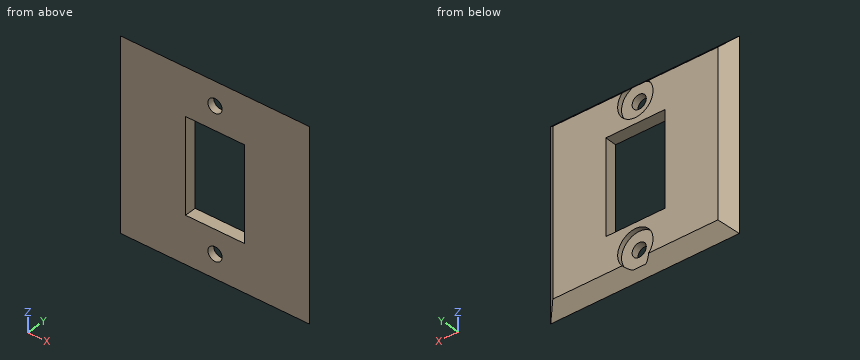
```python
from build123d import *

# Parameters (mm, degrees)
SKETCH1_W           = 40
SKETCH1_H           = 40
SKETCH1_W_2         = 12.5
SKETCH1_H_2         = 20
BOSS_EXTRUDE1_DEPTH = 2.5
SKETCH2_R           = 1.5
CUT_EXTRUDE1_DEPTH  = 10
SKETCH3_R           = 3.75
CUT_EXTRUDE2_DEPTH  = 1
CHAMFER1_SIZE       = 2.5


with BuildPart() as part:
    # Sketch1 → Boss-Extrude1 (new body)
    with BuildSketch(Plane(origin=(0, 0, 0), x_dir=(1, 0, 0), z_dir=(0, 1, 0))):
        Rectangle(SKETCH1_W, SKETCH1_H)
        Rectangle(SKETCH1_W_2, SKETCH1_H_2, mode=Mode.SUBTRACT)
    extrude(amount=BOSS_EXTRUDE1_DEPTH)

    # Sketch2 → Cut-Extrude1 (cut)
    with BuildSketch(Plane(origin=(0, 2.5, 0), x_dir=(1, 0, 0), z_dir=(0, 1, 0))):
        with Locations(Location((0, 15, 0), (0, 0, 270))):
            Circle(SKETCH2_R)
        with Locations(Location((0, -15, 0), (0, 0, 270))):
            Circle(SKETCH2_R)
    extrude(amount=-CUT_EXTRUDE1_DEPTH, mode=Mode.SUBTRACT)

    # Sketch3 → Cut-Extrude2 (cut)
    with BuildSketch(Plane(origin=(0, 2.5, 0), x_dir=(1, 0, 0), z_dir=(0, 1, 0))):
        with Locations(Location((0, 15, 0), (0, 0, 270))):
            Circle(SKETCH3_R)
        with Locations(Location((0, -15, 0), (0, 0, 270))):
            Circle(SKETCH3_R)
    extrude(amount=-CUT_EXTRUDE2_DEPTH, mode=Mode.SUBTRACT)

    # Chamfer1
    # the kernel refuses this chamfer: 2.5 mm, written as the material it takes off along each edge
    with BuildSketch(Plane(origin=(20, 2.5, -26.42920747), x_dir=(0.027495876610586317, -0.9996219169112968, 0), z_dir=(0, 0, 1)), Plane(origin=(-26.42920747, 2.5, -20), x_dir=(0, -0.9996219169112968, -0.027495876610586317), z_dir=(1, 0, 0)), Plane(origin=(-20, 2.5, 26.42920747), x_dir=(-0.027495876610586317, -0.9996219169112968, 0), z_dir=(0, 0, -1))) as chamfer1_piece_1:
        Polygon((CHAMFER1_SIZE * 0.999621916911, -CHAMFER1_SIZE * 0.0274958766106), (-CHAMFER1_SIZE * 0.0274958766106, -CHAMFER1_SIZE * 0.999621916911), (0, 0), align=None)
    extrude(amount=52.85841494, mode=Mode.SUBTRACT)
    with BuildSketch(Plane(origin=(26.42920747, 2.5, 20), x_dir=(0, 0.027495876610586317, -0.9996219169112968), z_dir=(-1, 0, 0))) as chamfer1_piece_2:
        Polygon((CHAMFER1_SIZE * 0.999621916911, CHAMFER1_SIZE * 0.0274958766106), (-CHAMFER1_SIZE * 0.0274958766106, CHAMFER1_SIZE * 0.999621916911), (0, 0), align=None)
    extrude(amount=52.85841494, mode=Mode.SUBTRACT)


solid = part.part
```
Source: CAD feature listing. Evaluate the final solid. Frame: model axes, mm. Give positions to 0.01 mm unless a question says otherwise; leave off trailing zeros. Write each loop counter-clockwise with the first axis right and the second up, starting at its lowest first coordinate (ties: lowest second). Pieces come first, ordered by that corner, then holes.
1. First-contact query: pin 1 (10 mm diameter, centred on x = 0, z = -15, fed in from +Y); pin 2 (6 mm diameter, centred on x = 0.5, z = 15.5, fed in from +Y); pin 3 (1.2 mm diameter, centred on x = -2.5, y = 1.5, fed in from -Z). Flat tips, straight axial feed; report the tip coordinate or a pass-through.
2. Material intervals for line 1 along Z through (x, y) = (0, 1.9); line 2 along X through (y, z) = (1.5, 5); line 3 along Y through (x, z) = (2.5, -12.5), sorted ascending.
3. Section query C-C (y = 0.6). Return the cut outline in (x, z), then the cut area to 3 significant figures.
4. Section query D-D (z = 0). Return the cut outline in (x, y).
5. Section query A-A (z = 15). Return the cut outline in (x, y).
6. Section query B-B (x = 0). Return the cut outline in (y, z), then the cut area to 4 significant figures.
Output values:
1. pin 1: stops at y = 2.5
1. pin 2: stops at y = 1.5
1. pin 3: stops at z = -19.1
2. line 1: z = -11.25 to -10, 10 to 11.25
2. line 2: x = -18.5 to -6.25, 6.25 to 18.5
2. line 3: y = 0 to 1.5
3. outline: (-19.4, -19.4) - (19.4, -19.4) - (19.4, 19.4) - (-19.4, 19.4) - close; hole (-6.25, -10) - (6.25, -10) - (6.25, 10) - (-6.25, 10) - close; hole circle Ø3 at (0, -15); hole circle Ø3 at (0, 15)
3. area: 1,240 mm2
4. outline: (-20, 0) - (-6.25, 0) - (-6.25, 2.5) - (-17.5, 2.5) - close; (6.25, 0) - (20, 0) - (17.5, 2.5) - (6.25, 2.5) - close
5. outline: (-20, 0) - (-1.5, 0) - (-1.5, 1.5) - (-3.75, 1.5) - (-3.75, 2.5) - (-17.5, 2.5) - close; (1.5, 0) - (20, 0) - (17.5, 2.5) - (3.75, 2.5) - (3.75, 1.5) - (1.5, 1.5) - close
6. outline: (0, -20) - (1.5, -18.5) - (1.5, -16.5) - (0, -16.5) - close; (0, -13.5) - (1.5, -13.5) - (1.5, -11.25) - (2.5, -11.25) - (2.5, -10) - (0, -10) - close; (0, 10) - (2.5, 10) - (2.5, 11.25) - (1.5, 11.25) - (1.5, 13.5) - (0, 13.5) - close; (0, 16.5) - (1.5, 16.5) - (1.5, 18.5) - (0, 20) - close
6. area: 21.25 mm2
